Could you check a few things on this drawing? It's one solid part, dimensions in mm from its lowest x, y, z. A direction names the side the tool comes from. Round coordinates to 2 decimals unless told otherwise and drop trailing zeros. Loops run counter-clockwise (first coordinate to the right, second up) from the corner with the lowest first, then second, coordinate; pieces in that order, holes last. Notation, with made-up numbers: M 83.5,-17 L 116.5,-17 A16 ccw 116.5,-2 Z; hole C 20,7 d8. An arc over 180 degrees is marked long. Use a Markdown table: item, result. Add a question column.
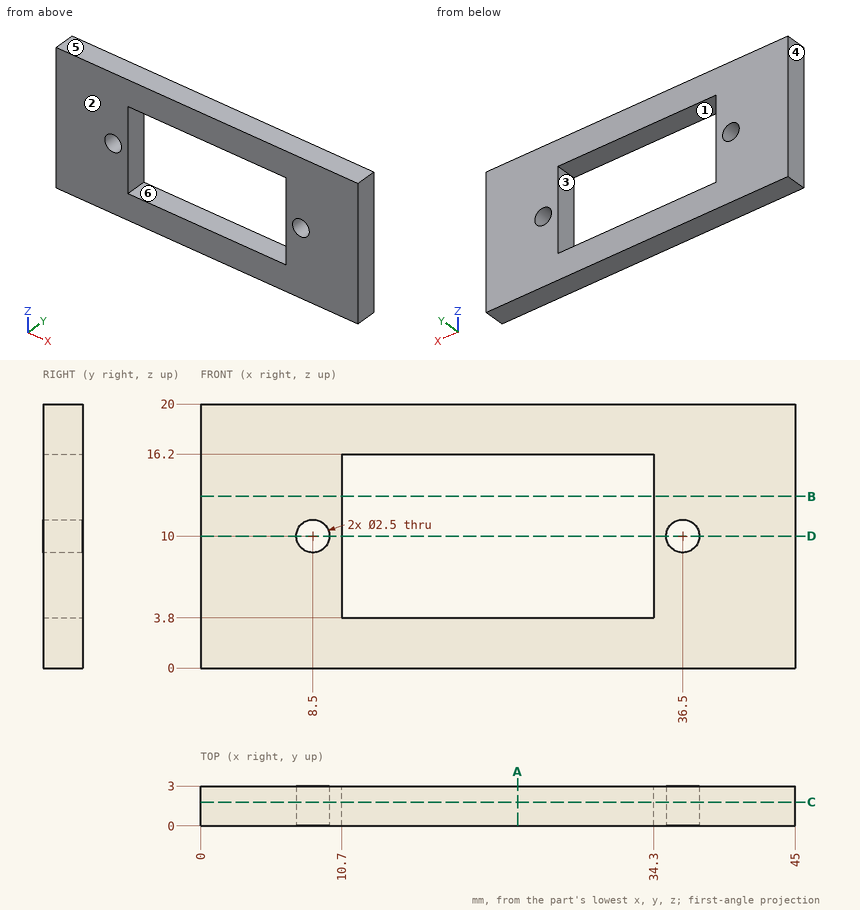
(1) If I drill on probe 1 along X at (y, z) = (0.85, 10); probe 2 along Z at (x, y) = (18.5, 0.75); probe 3 along Z at (x, y) = (36.5, 2.25), over which ranges is the centre line in solid material (lowest first)? Write a range as [from, to].
(2) Suppose I cut it at B-B on z = 13. List the corners of the cut face in (x, y) for me, and give its area (3 significant figures).
(3) On a 3-axis mill with a long thin cutter (end or side, diameter ignored), from which of +Z, -Z, +X, -X, +Y, -Y can I reach the whole of each face in a straight line? I mean the marked faces 1 and 2. Say none if no direction works.
(4) I'm going to push a flat-ended pin straight in: pin 1 (1.5 mm diameter, centred on x = 36.5, z = 10, fed in from -Y). Where does the tip first touch, or does it pass through?
(5) Suppose I cut it at D-D on z = 10. List the corners of the cut face in (x, y) for me, and give its area (3 significant figures).
(6) Suppose I cut it at C-C on y = 1.8. List the corners of the cut face in (x, z) for me.
(7) Thinking about a two-plate mould opening in Z: for the marked faces 3, 4, 5 and 6, which applies, released by +Z, released by -Z, zero draft, split by the parting line, or undercut?
(8) Suppose I cut it at A-A on x = 24. List the corners of the cut face in (y, z) for me, and give its area (3 significant figures).
Results below:
| question | item | result |
|---|---|---|
| 1 | probe 1 | x = [0, 7.25], [9.75, 10.7], [34.3, 35.25], [37.75, 45] |
| 1 | probe 2 | z = [0, 3.8], [16.2, 20] |
| 1 | probe 3 | z = [0, 8.75], [11.25, 20] |
| 2 | outline | M 0,0 L 10.7,0 L 10.7,3 L 0,3 Z; M 34.3,0 L 45,0 L 45,3 L 34.3,3 Z |
| 2 | area | 64.2 mm² |
| 3 | face 1 | +Y, -Y |
| 3 | face 2 | +Z, -Z, +X, -X, -Y |
| 4 | pin 1 | passes through |
| 5 | outline | M 0,0 L 7.25,0 L 7.25,3 L 0,3 Z; M 9.75,0 L 10.7,0 L 10.7,3 L 9.75,3 Z; M 34.3,0 L 35.25,0 L 35.25,3 L 34.3,3 Z; M 37.75,0 L 45,0 L 45,3 L 37.75,3 Z |
| 5 | area | 49.2 mm² |
| 6 | outline | M 0,0 L 45,0 L 45,20 L 0,20 Z; hole C 8.5,10 d2.5; hole M 10.7,3.8 L 34.3,3.8 L 34.3,16.2 L 10.7,16.2 Z; hole C 36.5,10 d2.5 |
| 7 | face 3 | undercut |
| 7 | face 4 | zero draft |
| 7 | face 5 | released by +Z |
| 7 | face 6 | undercut |
| 8 | outline | M 0,0 L 3,0 L 3,3.8 L 0,3.8 Z; M 0,16.2 L 3,16.2 L 3,20 L 0,20 Z |
| 8 | area | 22.8 mm² |
